The listing builds one solid part. Answer for the finished solid, in the listing's coordinates (mm). A direction names the side the tool comes from. Coordinates: 2 decimals unless noted, no trailing zeros. Order: outer loops, then holes, each group sorted by start corner. A loop starts at its lowest first (then second) coordinate and runs counter-clockwise, first axis right, second up. Notation, with made-up numbers: (63.5, -35.5) -> (75.5, -35.5) arc R19 cw to (75.5, -19.5) -> close; hole circle Ø7 at (-33.75, 60.25). An arc over 180 degrees is marked (long way). Write item = value, one per line.
from build123d import *

# Parameters (mm, degrees)
F0_W            = 45
F0_H            = 45
F1_DEPTH        = 1500
F2_W            = 45
F2_H            = 500
F3_DEPTH        = 45
F5_DEPTH        = 5
F5_COPIES_COUNT = 3
F5_COPIES_PITCH = 400
F8_DEPTH        = 5
F11_DEPTH       = 5


# Not quite as in the source:
# - a pattern or mirror of a feature is missing from the dataset's text; its kind, count and spacing are read off the source's solid


with BuildPart() as f1:
    # F0 (on Front) → F1 (new body, symmetric)
    with BuildSketch(Plane.XZ):
        Rectangle(F0_W, F0_H)
    extrude(amount=F1_DEPTH, both=True)

    # F2 (on face) → F3 (cut, through all)
    with BuildSketch(Plane.XY.offset(22.5)):
        Polygon((22.5, -1000), (-22.5, -955), (-22.5, -1500), (22.5, -1500), align=None)
        with Locations((0, 1250)):
            Rectangle(F2_W, F2_H)
    extrude(amount=-F3_DEPTH, mode=Mode.SUBTRACT)

    # F4 (on Front) → F5 (cut, symmetric)
    with BuildSketch(Plane.XZ):
        Polygon((22.5, 22.5), (-22.5, 22.5), (-22.5, 7.5), (7.5, 7.5), (7.5, -22.5), (22.5, -22.5), align=None)
    f5 = extrude(amount=F5_DEPTH, both=True, mode=Mode.SUBTRACT)

    # F5_copies: F5 ×3
    with Locations(*[(0, i * F5_COPIES_PITCH, 0) for i in range(1, F5_COPIES_COUNT)]):
        add(f5, mode=Mode.SUBTRACT)

    # F7 (on offset) → F8 (cut, symmetric)
    with BuildSketch(Plane.XZ.offset(400)):
        Polygon((-22.5, 22.5), (-22.5, 7.5), (7.5, 7.5), (7.5, -22.5), (22.5, -22.5), (22.5, 22.5), align=None)
    extrude(amount=F8_DEPTH, both=True, mode=Mode.SUBTRACT)

    # F10 (on offset) → F11 (cut, symmetric)
    with BuildSketch(Plane.XZ.offset(800)):
        Polygon((-22.5, 22.5), (-22.5, 7.5), (7.5, 7.5), (7.5, -22.5), (22.5, -22.5), (22.5, 22.5), align=None)
    extrude(amount=F11_DEPTH, both=True, mode=Mode.SUBTRACT)


solid = f1.part
Q1. Find the intervals of material crossed by line 1 along Y through (x, z) = (3, 19); line 2 along Y through (x, z) = (9, -8.5); line 3 along Y through (x, z) = (-12, -1.5), in increasing order.
The answers:
line_1 = -980.5 to -805, -795 to -405, -395 to -5, 5 to 395, 405 to 795, 805 to 1000
line_2 = -986.5 to -805, -795 to -405, -395 to -5, 5 to 395, 405 to 795, 805 to 1000
line_3 = -965.5 to 1000
Q2. The mould has two halves that part along Y. Classify faces 1 (the face through (0.3, -977.8, 0.3)), 2 (the face through (-22.5, 9, 0)), 3 (the face through (5, -405, 10)), 4 (the face through (5, 795, 10)): released by +Y, released by -Y, zero draft, split by the parting line, or undercut.
The answers:
face_1 = released by -Y
face_2 = zero draft
face_3 = undercut
face_4 = undercut
Q3. Each of these flat-tipped pins is pushed along its axis until it touches: pin 1 Ø8 at (x, z) = (10.5, 0) entering from -Y; pin 2 Ø3 at (x, y) = (-13, -800) entering from +Z; pin 3 Ø11 at (y, z) = (-798.5, -4.5) entering from +X; pin 4 Ø10 at (x, z) = (-15.5, 5) entering from -Y. Where does it stop, or does it pass through?
The answers:
pin_1 = -992
pin_2 = 7.5
pin_3 = 22.5
pin_4 = -967
Q4. Section A-A, the plane x = -11 is taken. Give the vertices of the cut face in (y, z).
The answers:
outline = (-966.5, -22.5) -> (1000, -22.5) -> (1000, 22.5) -> (805, 22.5) -> (805, 7.5) -> (795, 7.5) -> (795, 22.5) -> (405, 22.5) -> (405, 7.5) -> (395, 7.5) -> (395, 22.5) -> (5, 22.5) -> (5, 7.5) -> (-5, 7.5) -> (-5, 22.5) -> (-395, 22.5) -> (-395, 7.5) -> (-405, 7.5) -> (-405, 22.5) -> (-795, 22.5) -> (-795, 7.5) -> (-805, 7.5) -> (-805, 22.5) -> (-966.5, 22.5) -> close
Q5. Section B-B, the plane z = -1.5 is taken. Give the vertices of the cut face in (x, y), plus the area to 3 significant figures.
The answers:
outline = (-22.5, -955) -> (22.5, -1000) -> (22.5, -805) -> (7.5, -805) -> (7.5, -795) -> (22.5, -795) -> (22.5, -405) -> (7.5, -405) -> (7.5, -395) -> (22.5, -395) -> (22.5, -5) -> (7.5, -5) -> (7.5, 5) -> (22.5, 5) -> (22.5, 395) -> (7.5, 395) -> (7.5, 405) -> (22.5, 405) -> (22.5, 795) -> (7.5, 795) -> (7.5, 805) -> (22.5, 805) -> (22.5, 1000) -> (-22.5, 1000) -> close
area = 88,200 mm2
Q6. A tool of negligible diameter and unlimited length cuts with its end or side. For faces 5 (the face through (5, -5, 10)), 6 (the face through (22.5, 597, 0)), from which of +Z, -Z, +X, -X, +Y, -Y can it reach the whole face along a straight path? Write none if from no direction.
The answers:
face_5 = +Z, +X
face_6 = +Z, -Z, +X, +Y, -Y
